Job drawing, mm, ordinate dimensions from the low corner. One solid piece. A direction names the side the tool comes from. Coordinates: 2 decimals unless noted, no trailing zeros. Order: outer loops, then holes, each group sorted by start corner. A loop starts at its lowest first (then second) coordinate and runs counter-clockwise, first axis right, second up. Notation, with made-up numbers: (-27, 12) - (6, 12) arc R25 ccw to (6, 44) - close; hole circle Ø6 at (29, 52.25). An arc over 180 degrees is marked (long way). Write each question's results on one line, items separated by ' | '. Start each with the question number.
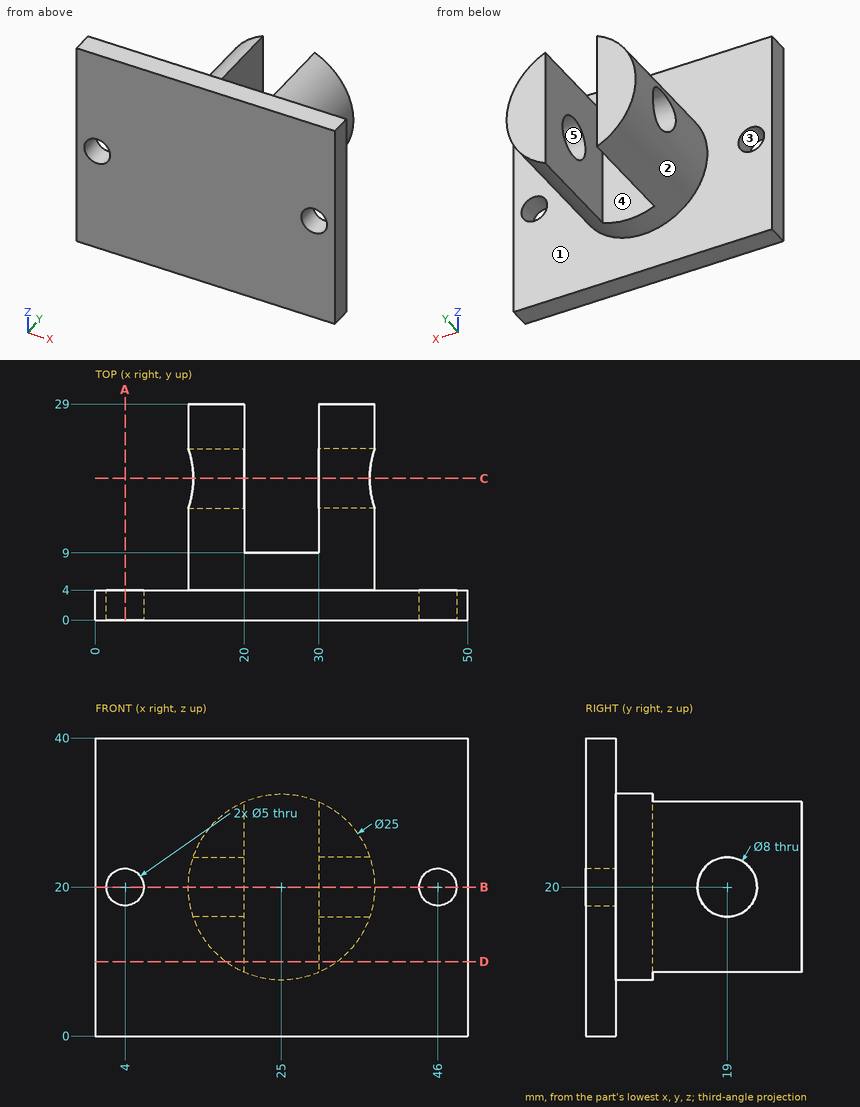
Item 1: Pull direction Z, two halves, no side cores. Call the marked faces 1, 2 and 3: released by +Z, released by -Z, zero draft, split by the parting line, or undercut.
Item 2: Flat gauge pins, fed straight in: P1, Ø5, axis at x = 23, z = 14.5, coming from the +Y side; P2, Ø1.5, axis at x = 40, z = 18.5, coming from the +Y side; P3, Ø4, axis at y = 18.5, z = 25, coming from the -X side; P4, Ø2, axis at x = 38, z = 8, coming from the -Y side. Where does each tip first touch, or does it go through?
Item 3: Slice it at D-D (z = 10). Write the cut outline in (x, y), then the cut area to 3 significant figures.
Item 4: Slice it at C-C (y = 19). Write the cut outline in (x, z), then the cut area to 3 significant figures.
Item 5: Which spindle directions (+Z, -Z, +X, -X, +Y, -Y) get a long thin tool onto all of the face, cutting with end or side? Do the marked faces 4 and 5. Say none if no direction does.
Item 6: Slice it at B-B (z = 20). Write the cut outline in (x, y), then the cut area to 3 significant figures.
Item 7: Slice it at A-A (x = 4). Write the cut outline in (y, z), then the cut area to 3 significant figures.
Item 8: Probe probe 1 along Y at (x, z) = (15.5, 20); probe 2 along Z at (x, y) = (4, 1); probe 3 along X at (y, z) = (2.2, 20). List the from-to ranges inside material, lowest first.
Resolved:
1) face 1: zero draft | face 2: split by the parting line | face 3: undercut
2) P1: y = 9 | P2: y = 4 | P3: x = 13.01 | P4: y = 0
3) outline: (0, 0) - (50, 0) - (50, 4) - (32.5, 4) - (32.5, 29) - (30, 29) - (30, 9) - (20, 9) - (20, 29) - (17.5, 29) - (17.5, 4) - (0, 4) - close | area: 375 mm^2
4) outline: (13.16, 16) arc R12.5 ccw to (20, 8.54) - (20, 16) - close; (13.16, 24) - (20, 24) - (20, 31.46) arc R12.5 ccw to start; (30, 8.54) arc R12.5 ccw to (36.84, 16) - (30, 16) - close; (30, 24) - (36.84, 24) arc R12.5 ccw to (30, 31.46) - close | area: 131 mm^2
5) face 4: +Z, -Z, +Y | face 5: +X, -X
6) outline: (0, 0) - (1.5, 0) - (1.5, 4) - (0, 4) - close; (6.5, 0) - (43.5, 0) - (43.5, 4) - (37.5, 4) - (37.5, 15) - (30, 15) - (30, 9) - (20, 9) - (20, 15) - (12.5, 15) - (12.5, 4) - (6.5, 4) - close; (12.5, 23) - (20, 23) - (20, 29) - (12.5, 29) - close; (30, 23) - (37.5, 23) - (37.5, 29) - (30, 29) - close; (48.5, 0) - (50, 0) - (50, 4) - (48.5, 4) - close | area: 465 mm^2
7) outline: (0, 0) - (4, 0) - (4, 17.5) - (0, 17.5) - close; (0, 22.5) - (4, 22.5) - (4, 40) - (0, 40) - close | area: 140 mm^2
8) probe 1: 0 to 15, 23 to 29 | probe 2: 0 to 17.5, 22.5 to 40 | probe 3: 0 to 1.5, 6.5 to 43.5, 48.5 to 50
